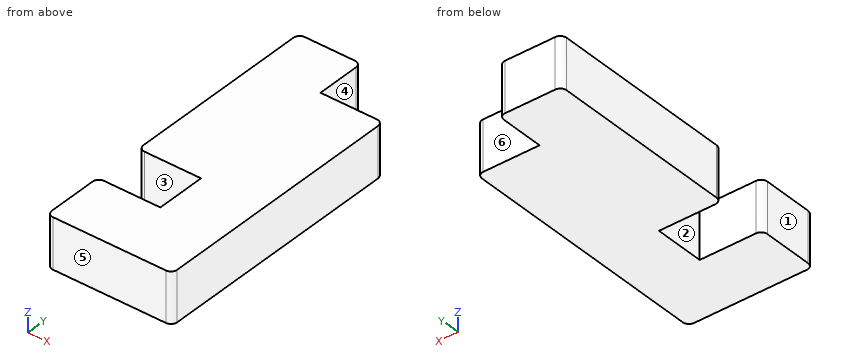
from build123d import *

# Parameters (mm, degrees)
BOSS_EXTRUDE1_DEPTH = 8


with BuildPart() as part:
    # Sketch1 → Boss-Extrude1 (new body)
    with BuildSketch(Plane.XY):
        with BuildLine():
            Line((1, 0), (19, 0))
            ThreePointArc((19, 0), (19.707106781, 0.292893219), (20, 1))
            Line((20, 1), (20, 40.5))
            ThreePointArc((20, 40.5), (19.707106781, 41.207106781), (19, 41.5))
            Line((19, 41.5), (10, 41.5))
            Line((10, 41.5), (10, 48.5))
            ThreePointArc((10, 48.5), (9.707106781, 49.207106781), (9, 49.5))
            Line((9, 49.5), (1, 49.5))
            ThreePointArc((1, 49.5), (0.292893219, 49.207106781), (0, 48.5))
            Line((0, 48.5), (0, 19))
            ThreePointArc((0, 19), (0.292893219, 18.292893219), (1, 18))
            Line((1, 18), (10, 18))
            Line((10, 18), (10, 10))
            Line((10, 10), (1, 10))
            ThreePointArc((1, 10), (0.292893219, 9.707106781), (0, 9))
            Line((0, 9), (0, 1))
            ThreePointArc((0, 1), (0.292893219, 0.292893219), (1, 0))
        make_face()
    extrude(amount=BOSS_EXTRUDE1_DEPTH)


solid = part.part
Verification items for the finished model (mm, model axes). Face numbers are marked on the shaded views. A direction names the side the tool comes from. Give positions to 0.01 mm unless a question says otherwise; leave off trailing zeros. Write each loop counter-clockwise with the first axis right and the second up, starting at its lowest first coordinate (ties: lowest second). Pieces come first, ordered by that corner, then holes. Notation, with made-up numbers: M -29,28.25 L -6,28.25 A29 cw -6,56.25 Z; hole C 51,68 d11. An arc over 180 degrees is marked long. Put each result on its own line as item: value. Start each with the question number.
1. Section check C-C (y = 17.5). Record the cut outline in (x, z), and give its area (3 significant figures).
2. Draft check along Y on the marked faces 3, 4, 5 and 6. Enter one of: +Y half, -Y half, draft (parallel to the pull), parting line (faces both ways), or undercut.
3. Set-up check for the marked faces 1 and 2: record each of +Z, -Z, +X, -X, +Y, -Y from which the full face is reachable in a straight line by a thin tool's end or side.
4. Scan lines: line 1 along Y through (x, z) = (9, 1.25); line 2 along X through (y, z) = (47.5, 5.75); line 3 along X through (y, z) = (12, 3.25). Record each from-to range of solid material in increasing order. Write a range as [from, to].
5. Go/stop test with flat-tipped pins: pin 1 Ø2.5 at (y, z) = (14.5, 6) entering from -X; pin 2 Ø2.5 at (x, z) = (15.5, 5) entering from +Y. Record where each tip stops, or that it passes through.
6. Section check B-B (z = 2.5). Record the cut outline in (x, y), and give its area (4 significant figures).
7. Section check D-D (x = 11.5). Record the cut outline in (y, z), and give its area (3 significant figures).
8. Section check A-A (x = 7.25). Record the cut outline in (y, z).
Answer list:
1. outline: M 10,0 L 20,0 L 20,8 L 10,8 Z
1. area: 80.0 mm2
2. face 3: undercut
2. face 4: draft
2. face 5: -Y half
2. face 6: +Y half
3. face 1: +Z, -Z, -X, +Y, -Y
3. face 2: +Z, -Z, -X
4. line 1: [0, 10], [18, 49.5]
4. line 2: [0, 10]
4. line 3: [10, 20]
5. pin 1: x = 10
5. pin 2: y = 41.5
6. outline: M 0,1 A1 ccw 1,0 L 19,0 A1 ccw 20,1 L 20,40.5 A1 ccw 19,41.5 L 10,41.5 L 10,48.5 A1 ccw 9,49.5 L 1,49.5 A1 ccw 0,48.5 L 0,19 A1 ccw 1,18 L 10,18 L 10,10 L 1,10 A1 ccw 0,9 Z
6. area: 828.5 mm2
7. outline: M 0,0 L 41.5,0 L 41.5,8 L 0,8 Z
7. area: 332 mm2
8. outline: M 0,0 L 10,0 L 10,8 L 0,8 Z; M 18,0 L 49.5,0 L 49.5,8 L 18,8 Z
